The listing builds one solid part. Answer for the finished solid, in the listing's coordinates (mm). A direction names the side the tool comes from. Give positions to 0.01 mm unless a question says otherwise; leave off trailing zeros. Write each loop counter-clockwise with the first axis right and the second up, starting at its lowest first coordinate (ties: lowest second). Pieces come first, ordered by that corner, then holes. Notation, with made-up numbers: M -28,-31.5 L -20,-31.5 A22 cw -20,-19.5 Z; hole C 30,-2 d6. An arc over 180 degrees is marked long. Return JSON: item names as keys, results as strings.
from build123d import *

# Parameters (mm, degrees)
SKETCH2_R               = 12.5
BOSS_EXTRUDE1_DEPTH     = 2.5
BOSS_EXTRUDE2_DEPTH     = 5
SKETCH5_W               = 50
SKETCH5_H               = 35
BOSS_EXTRUDE3_DEPTH     = 15
CUT_EXTRUDE1_DEPTH      = 171.878020085
CUT_EXTRUDE1_DEPTH_BACK = 171.878020085


with BuildPart() as part:
    # Sketch2 → Boss-Extrude1 (new body)
    with BuildSketch(Plane.XY):
        Circle(SKETCH2_R)
        with BuildLine():
            ThreePointArc((1.389019438, -1.575), (0, 2.1), (-1.389019438, -1.575))
            Line((-1.389019438, -1.575), (0, -1.575))
            Line((0, -1.575), (1.389019438, -1.575))
        make_face(mode=Mode.SUBTRACT)
    extrude(amount=BOSS_EXTRUDE1_DEPTH)

    # Sketch4 → Boss-Extrude2 (add)
    with BuildSketch(Plane.XY.offset(2.5)):
        Polygon((-5, -162.170582253), (5, -162.170582253), (5, -4.038316712), (0, -4.038316712), (-5, -4.038316712), align=None)
    extrude(amount=BOSS_EXTRUDE2_DEPTH)

    # Sketch5 → Boss-Extrude3 (add)
    with BuildSketch(Plane(origin=(5, 0, 0), x_dir=(0, 0, -1), z_dir=(1, 0, 0))):
        with Locations((-5, -144.670582253)):
            Rectangle(SKETCH5_W, SKETCH5_H)
    extrude(amount=BOSS_EXTRUDE3_DEPTH)

    # Sketch6 → Cut-Extrude1 (cut, two sides: drawn at the far end of the back side and taken through both)
    with BuildSketch(Plane(origin=(0, 0, -20), x_dir=(-1, 0, 0), z_dir=(0, 0, -1)).offset(-CUT_EXTRUDE1_DEPTH_BACK)):
        with BuildLine():
            Line((-20, -127.170582253), (-5, -127.170582253))
            ThreePointArc((-5, -127.170582253), (-9.438654014, -145.982587676), (-20, -162.170582253))
            Line((-20, -162.170582253), (-20, -127.170582253))
        make_face()
    extrude(amount=CUT_EXTRUDE1_DEPTH + CUT_EXTRUDE1_DEPTH_BACK, mode=Mode.SUBTRACT)


solid = part.part
Item 1: A cutting plane is placed at B-B, the plane z = 5. Write down the section's boundary in (x, y).
Geometry results:
{"outline": "M -5,-162.17 L 20,-162.17 A56.08 cw 5,-127.17 L 5,-4.04 L -5,-4.04 Z"}
Item 2: Given pin 1 Ø10 at (x, y) = (-6.5, -13.5) entering from +Z; pin 2 Ø3 at (x, y) = (0.5, -83.5) entering from -Z; pin 3 Ø12 at (x, y) = (-2.5, 6) entering from +Z; pin 4 Ø6 at (x, z) = (-2.5, -4.5) entering from -Y, each flat-ended and moving along its own axis, determine where each tip first touches the part or whether it passes through.
Geometry results:
{"pin 1": "stops at z = 7.5", "pin 2": "stops at z = 2.5", "pin 3": "stops at z = 2.5", "pin 4": "passes through"}
Item 3: A cutting plane is placed at C-C, the plane y = -31. Write down the section's boundary in (x, z), plus the area to 3 significant figures.
Geometry results:
{"outline": "M -5,2.5 L 5,2.5 L 5,7.5 L -5,7.5 Z", "area": "50.0 mm2"}
Item 4: A cutting plane is placed at D-D, the plane x = 16. Write down the section's boundary in (y, z).
Geometry results:
{"outline": "M -162.17,-20 L -157.38,-20 L -157.38,30 L -162.17,30 Z"}
Item 5: Determine the mould class of faces 4 (the flat face through (13, -162.171, 5)), 5 (the cylindrical face through (0.07, 2.1, 1.23)), 6 (the flat face through (0, -4.038, 5)), 7 (the flat face through (9, -153, 30)) for opening direction Y: +Y half, -Y half, draft (parallel to the pull), parting line (faces both ways), or undercut.
Geometry results:
{"face 4": "-Y half", "face 5": "undercut", "face 6": "+Y half", "face 7": "draft"}
Item 6: Find the intervals of material crossed by line 1 (X direction, y = 0, z = 1); line 2 (Y direction, x = 0, z = 1) (3 decimals); line 3 (Z direction, x = 1.5, y = -131), in increasing order.
Geometry results:
{"line 1": "x = -12.5 to -2.1, 2.1 to 12.5", "line 2": "y = -12.5 to -1.575, 2.1 to 12.5", "line 3": "z = 2.5 to 7.5"}
Item 7: A cutting plane is placed at A-A, the plane y = 0. Write down the section's boundary in (x, z).
Geometry results:
{"outline": "M -12.5,0 L -2.1,0 L -2.1,2.5 L -12.5,2.5 Z; M 2.1,0 L 12.5,0 L 12.5,2.5 L 2.1,2.5 Z"}
Item 8: Which of the six approach directions +Z, -Z, +X, -X, +Y, -Y give full straight-line access (tool end or side, diameter ignored) to faces 1 (the flat face through (0, -3, 0)), 2 (the flat face through (0, -82, 7.5)), 3 (the flat face through (0, -86, 2.5))?
Geometry results:
{"face 1": "-Z, +X, -X, +Y", "face 2": "+Z, -X, +Y, -Y", "face 3": "-Z, -X, -Y"}
